Autodesk Inventor part; units mm, degrees
ref_plane "YZ Plane" through (0, 0, 0) normal (1, 0, 0) x (0, 1, 0)
ref_plane "XZ Plane" through (0, 0, 0) normal (0, 1, 0) x (-1, 0, 0)
ref_plane "XY Plane" through (0, 0, 0) normal (0, 0, 1) x (1, 0, 0)
sketch "スケッチ1" plane through (0, 0, 0) normal (0, 1, 0) x (-1, 0, 0)
  circle A0 centre (0, 0) radius 10
  line L0 (0, 10) -> (-10, 10)
  line L1 (-10, 10) -> (-10, -10)
  line L2 (-10, -10) -> (10, -10)
  line L3 (10, -10) -> (10, 0)
  dimension "d0" = 20
  dimension "d1" = 10
  dimension "d2" = 10
extrude "押し出し1" add sketch "スケッチ1" along normal blind 77
sketch "スケッチ2" plane through (0, 0, 10) normal (0, 0, 1) x (1, 0, 0)
  line L0 (0, 0) -> (0, 77)
  line L1 (0, 77) -> (10, 77)
  line L2 (10, 77) -> (10, 0)
  line L3 (10, 0) -> (0, 0)
extrude "押し出し2" cut sketch "スケッチ2" against normal blind 1
sketch "スケッチ3" plane through (-10, 0, -10) normal (-1, 0, 0) x (0, 0, 1)
  line L0 (0, 77) -> (10, 77)
  line L1 (10, 0) -> (10, 77)
  line L2 (10, 0) -> (0, 0)
  line L3 (0, 0) -> (0, 77)
extrude "押し出し3" cut sketch "スケッチ3" against normal blind 1
sketch "スケッチ4" plane through (0, 0, 9) normal (0, 0, 1) x (1, 0, 0)
  line L0 (0, 77) -> (10, 77)
  line L1 (10, 77) -> (10, 0)
  line L2 (10, 0) -> (0, 0)
  point P0 (5, 72)
  point P1 (5, 5)
  dimension "d9" = 5
  dimension "d10" = 5
  dimension "d11" = 5
hole "穴1" at (5, 72, 9) at (5, 5, 9) direction (0, 0, -1) diameter 5 depth 6
sketch "スケッチ5" plane through (0, 0, 0) normal (0, 1, 0) x (1, 0, 0)
  point P0 (0, 0)
hole "穴2" at (0, 0, 0) direction (0, 1, 0) diameter 5 depth 6
sketch "スケッチ6" plane through (-9, 0, -10) normal (-1, 0, 0) x (0, 0, 1)
  line L0 (0, 0) -> (0, 77)
  line L1 (0, 77) -> (10, 77)
  line L2 (10, 0) -> (0, 0)
  point P0 (5, 72)
  point P1 (5, 5)
  dimension "d26" = 5
  dimension "d27" = 5
  dimension "d28" = 5
  dimension "d29" = 5
hole "穴3" at (-9, 72, -5) at (-9, 5, -5) direction (1, 0, 0) diameter 5 depth 6
sketch "スケッチ7" plane through (0, 77, 0) normal (0, 1, 0) x (1, 0, 0)
  circle A0 centre (0, 0) radius 3
  dimension "d37" = 6
extrude "押し出し4" cut sketch "スケッチ7" against normal blind 6
chamfer "面取り1" distance 3 angle 45 1 edges at (-3, 77, 0)
fillet "フィレット1" radius 10 1 edges at (10, 38.5, -10)
properties part number "base6" material "ABS プラスチック"
Verification items for the finished model (mm, model axes). A direction names the side the tool comes from. Coordinates: 2 decimals unless noted, no trailing zeros. Loops run counter-clockwise (first coordinate to the right, second up) from the corner with the lowest first, then second, coordinate; pieces in that order, holes last. Notation, with made-up numbers: (59.25, -34) -> (94.25, -34) arc R28 cw to (94.25, -13) -> close; hole circle Ø3 at (68, 23.25). An arc over 180 degrees is marked (long way). Put each result on its own line as item: value.
1. Section check A-A, the plane y = 72. Record the boundary of the cut face in (x, z), then the cut area to 3 significant figures.
Result set:
outline: (-10, 0) -> (-9, 0) -> (-9, -2.5) -> (-3, -2.5) -> (-3, -7.5) -> (-9, -7.5) -> (-9, -10) -> (0, -10) arc R10 ccw to (10, 0) -> (10, 9) -> (7.5, 9) -> (7.5, 3) -> (2.5, 3) -> (2.5, 9) -> (0, 9) -> (0, 10) arc R10 ccw to start; hole circle Ø6 at (0, 0)
area: 249 mm^2
2. Mould release check, pull along Y, two halves, no side actions. Record for faces 4 (the face through (-5.958, 4.249, -2.615)), 5 (the face through (-6.99, 37.96, 7.15)), 6 (the face through (-2, 0, -2)), 7 (the face through (-3, 72, -5)): pulls with the +Y half, pulls with the -Y half, needs draft (parallel to the pull), parting line crosses it, or undercut.
Result set:
face 4: undercut
face 5: needs draft
face 6: pulls with the -Y half
face 7: undercut
3. Section check C-C, the plane y = 5. Record the boundary of the cut face in (x, z), then the cut area to 3 significant figures.
Result set:
outline: (-10, 0) -> (-9, 0) -> (-9, -2.5) -> (-3, -2.5) -> (-3, -7.5) -> (-9, -7.5) -> (-9, -10) -> (0, -10) arc R10 ccw to (10, 0) -> (10, 9) -> (7.5, 9) -> (7.5, 3) -> (2.5, 3) -> (2.5, 9) -> (0, 9) -> (0, 10) arc R10 ccw to start; hole circle Ø5 at (0, 0)
area: 257 mm^2
4. Section check B-B, the plane x = 6.75. Record the boundary of the cut face in (y, z), then the cut area to 3 significant figures.
Result set:
outline: (0, -7.38) -> (77, -7.38) -> (77, 9) -> (73.79, 9) -> (73.79, 3) -> (70.21, 3) -> (70.21, 9) -> (6.79, 9) -> (6.79, 3) -> (3.21, 3) -> (3.21, 9) -> (0, 9) -> close
area: 1,220 mm^2
5. Thickness scan on line 1 (Y direction, x = -7.7, z = -5); line 2 (Z direction, x = -6.2, y = 72); line 3 (Y direction, x = -4, z = -3.25). Record the ranges inside material, lowest first.
Result set:
line 1: y = 0 to 2.5, 7.5 to 69.5, 74.5 to 77
line 2: z = -10 to -7.5, -2.5 to 7.85
line 3: y = 0 to 3.21, 6.79 to 70.21, 73.79 to 76.15
6. Gauge pin test, flat ends, axial feed: P1, Ø5.5, axis at x = 4.5, y = 5.5, coming from the +Z side; P2, Ø1.5, axis at x = -3, z = -2, coming from the +Y side; P3, Ø8, axis at x = 5, y = 5, coming from the -Z side. Record the tip position at first contact, or that the pin passes through.
Result set:
P1: stops at z = 9
P2: stops at y = 75.36
P3: stops at z = -9.95
7. Section check D-D, the plane y = 13.5. Record the boundary of the cut face in (x, z).
Result set:
outline: (-10, 0) -> (-9, 0) -> (-9, -10) -> (0, -10) arc R10 ccw to (10, 0) -> (10, 9) -> (0, 9) -> (0, 10) arc R10 ccw to start
8. Tool access check on faces 1 (the face through (-3, 5, -5)), 2 (the face through (2.44, 3.04, 0.54)), 3 (the face through (4.9, 74.5, 6)). Record the directions out of +Z, -Z, +X, -X, +Y, -Y that give a thin tool (end or side, any length) a straight path to the whole face; none if there is none.
Result set:
face 1: -X
face 2: -Y
face 3: +Z
